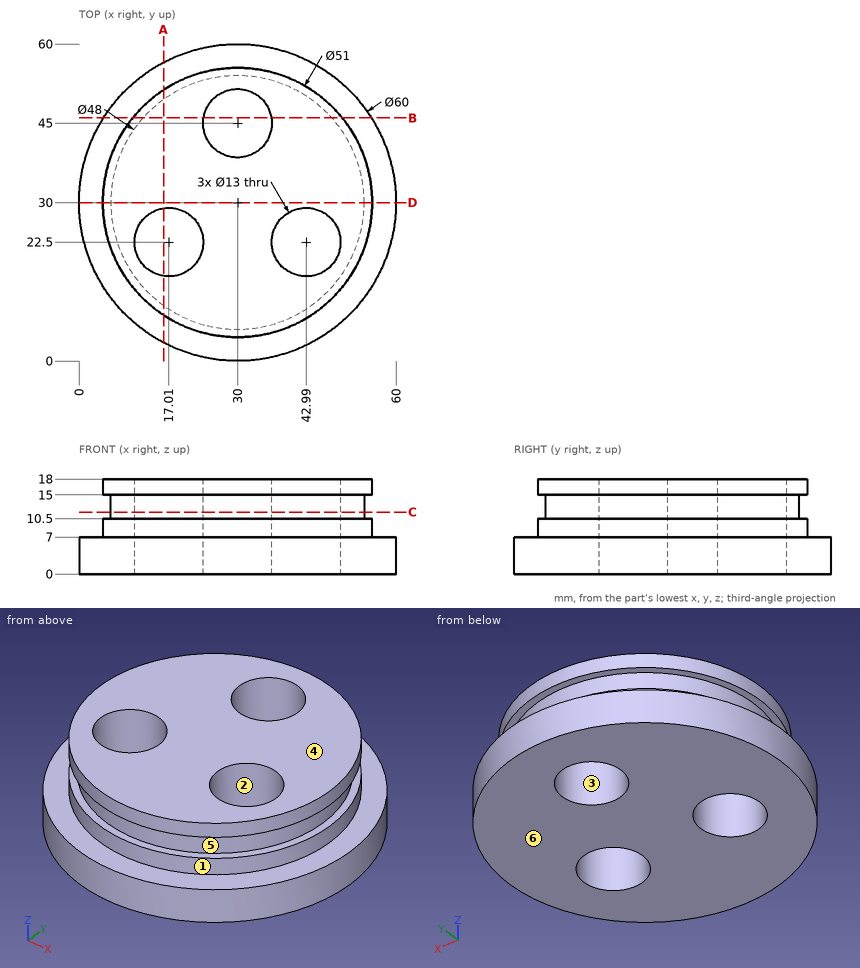
Verification items for this drawing (mm, ordinates from the low corner). A direction names the side the tool comes from. Give positions to 0.01 mm unless a question says otherwise; leave off trailing zeros. Loops run counter-clockwise (first coordinate to the right, second up) from the corner with the lowest first, then second, coordinate; pieces in that order, holes last. Notation, with made-up numbers: M 59,82 L 78,82 A13 cw 78,89 Z; hole C -19,-32 d5. An arc over 180 degrees is marked long. Answer as a JSON object with one key per item and string values. Group by question number.
Item 1: Access from +Z, -Z, +X, -X, +Y, -Y to the whole of each face (thin tool, end or side, straight path). Record for the marked faces 1 and 2.
Item 2: Sectioned sample at D-D on y = 30. Record the boundary of the cut face in (x, z).
Item 3: Sectioned sample at B-B on y = 46. Record the boundary of the cut face in (x, z) (1 decimal).
Item 4: Sectioned sample at A-A on x = 16. Record the boundary of the cut face in (y, z).
Item 5: Mould release check, pull along Z, two halves, no side actions. Record for the marked faces 3, 4, 5 and 6: pulls with the +Z half, pulls with the -Z half, needs draft (parallel to the pull), parting line crosses it, or undercut.
Item 6: Material ranges on L1, parallel to Z at x = 14, y = 11; L2, parallel to X at y = 22, z = 2.5; L3, parallel to Y at x = 30, z = 16.25, recorded low to high.
Item 7: Gauge pin test, flat ends, axial feed: pin 1 (21 mm diameter, centred on x = 17.01, y = 22.5, fed in from -Z); pin 2 (4 mm diameter, centred on y = 18, z = 6, fed in from +X) (1 decimal); pin 3 (1.5 mm diameter, centred on x = 14, z = 15.5, fed in from -Y). Record the tip position at first contact, or that the pin passes through.
Item 8: Sectioned sample at C-C on z = 11.75. Record the boundary of the cut face in (x, y).
Findings below:
{
 "1": {"face 1": "+Z", "face 2": "+Z, -Z"},
 "2": {"outline": "M 0,0 L 60,0 L 60,7 L 55.5,7 L 55.5,10.5 L 54,10.5 L 54,15 L 55.5,15 L 55.5,18 L 4.5,18 L 4.5,15 L 6,15 L 6,10.5 L 4.5,10.5 L 4.5,7 L 0,7 Z"},
 "3": {"outline": "M 4.6,0 L 23.6,0 L 23.6,18 L 10.1,18 L 10.1,15 L 12.1,15 L 12.1,10.5 L 10.1,10.5 L 10.1,7 L 4.6,7 Z; M 36.4,0 L 55.4,0 L 55.4,7 L 49.9,7 L 49.9,10.5 L 47.9,10.5 L 47.9,15 L 49.9,15 L 49.9,18 L 36.4,18 Z"},
 "4": {"outline": "M 3.47,0 L 16.08,0 L 16.08,18 L 8.69,18 L 8.69,15 L 10.51,15 L 10.51,10.5 L 8.69,10.5 L 8.69,7 L 3.47,7 Z; M 28.92,0 L 56.53,0 L 56.53,7 L 51.31,7 L 51.31,10.5 L 49.49,10.5 L 49.49,15 L 51.31,15 L 51.31,18 L 28.92,18 Z"},
 "5": {"face 3": "needs draft", "face 4": "pulls with the +Z half", "face 5": "undercut", "face 6": "pulls with the -Z half"},
 "6": {"L1": "0 to 10.5, 15 to 18", "L2": "1.09 to 10.53, 23.49 to 36.51, 49.47 to 58.91", "L3": "4.5 to 38.5, 51.5 to 55.5"},
 "7": {"pin 1": "z = 0", "pin 2": "x = 58.3", "pin 3": "y = 9.56"},
 "8": {"outline": "C 30,30 d48; hole C 17.01,22.5 d13; hole C 30,45 d13; hole C 42.99,22.5 d13"}
}
